```python
from build123d import *

# Parameters (mm, degrees)
SKETCH1_R           = 8.75
SKETCH1_R_2         = 6.75
BOSS_EXTRUDE1_DEPTH = 5.25
SKETCH2_R           = 10.25
SKETCH2_R_2         = 6.75
BOSS_EXTRUDE2_DEPTH = 1
CHAMFER1_SIZE       = 1.050311307
CHAMFER1_SIZE_2     = 1.5
CHAMFER2_SIZE       = 1
CHAMFER3_SIZE       = 0.5


with BuildPart() as part:
    # Sketch1 → Boss-Extrude1 (new, symmetric)
    with BuildSketch(Plane.XY):
        with Locations(Location((0, 0, 0), (0, 0, 180))):
            Circle(SKETCH1_R)
        with Locations(Location((0, 0, 0), (0, 0, 180))):
            Circle(SKETCH1_R_2, mode=Mode.SUBTRACT)
    extrude(amount=BOSS_EXTRUDE1_DEPTH, both=True)

    # Sketch2 → Boss-Extrude2 (add)
    with BuildSketch(Plane.XY.offset(5.25)):
        Circle(SKETCH2_R)
        with Locations(Location((0, 0, 0), (0, 0, 180))):
            Circle(SKETCH2_R_2, mode=Mode.SUBTRACT)
    boss_extrude2 = extrude(amount=BOSS_EXTRUDE2_DEPTH)

    # Mirror1: Boss-Extrude2 across plane
    add(boss_extrude2.mirror(Plane.XY))

    # Chamfer1
    # the kernel refuses this chamfer: 1.5, 1.050311307 mm, written as the material it adds along each edge
    with BuildSketch(Plane(origin=(0, 0, -5.25), x_dir=(-1, 0, 0), z_dir=(0, 1, 0))) as chamfer1_piece_1_section:
        Polygon((8.75, CHAMFER1_SIZE), (8.75 + CHAMFER1_SIZE_2, 0), (8.75, 0), align=None)
    chamfer1_piece_1 = revolve(axis=Axis((0, 0, -5.25), (0, 0, 1)), mode=Mode.PRIVATE)
    chamfer1_piece_1 = chamfer1_piece_1 & Plane(origin=(0, 0, -4.738052243), x_dir=(1, 0, 0), z_dir=(0, 0, 1)) * Cylinder(10.25, 42, mode=Mode.PRIVATE)
    add(chamfer1_piece_1)
    with BuildSketch(Plane(origin=(0, 0, 5.25), x_dir=(-1, 0, 0), z_dir=(0, 1, 0))) as chamfer1_piece_2_section:
        Polygon((8.75, -CHAMFER1_SIZE), (8.75 + CHAMFER1_SIZE_2, 0), (8.75, 0), align=None)
    chamfer1_piece_2 = revolve(axis=Axis((0, 0, 5.25), (0, 0, 1)), mode=Mode.PRIVATE)
    chamfer1_piece_2 = chamfer1_piece_2 & Plane(origin=(0, 0, 4.738052243), x_dir=(1, 0, 0), z_dir=(0, 0, -1)) * Cylinder(10.25, 42, mode=Mode.PRIVATE)
    add(chamfer1_piece_2)

    # Chamfer2
    chamfer2_edges = [part.edges().sort_by_distance(p)[0] for p in [
        (6.75, 0, 6.25),
        (6.75, 0, -6.25),
    ]]
    chamfer(chamfer2_edges, length=CHAMFER2_SIZE)

    # Chamfer3
    chamfer3_edges = [part.edges().sort_by_distance(p)[0] for p in [
        (-10.25, 0, 6.25),
        (-10.25, 0, -6.25),
    ]]
    chamfer(chamfer3_edges, length=CHAMFER3_SIZE)


solid = part.part
```
Design review of the part built by this model. Coordinates are the model's own, in mm. A direction names the side the tool comes from. Round coordinates to 2 decimals unless told otherwise and drop trailing zeros. Order: outer loops, then holes, each group sorted by start corner. A loop starts at its lowest first (then second) coordinate and runs counter-clockwise, first axis right, second up. Notation, with made-up numbers: M 78.5,40 L 111.5,40 A13 ccw 111.5,60 Z; hole C 70.5,53 d4. An arc over 180 degrees is marked long. Put each result on its own line as item: value.
Q1. Draft analysis for pull direction X (two halves, no side actions). For faces 1 (the face through (-7, -4, 6.25)), 2 (the face through (1.46, 6.59, 0.07)), 3 (the face through (-2.222, -10.006, -5.496)), state which applies: released by +X, released by -X, zero draft, split by the parting line, or undercut.
Reported:
face 1: zero draft
face 2: undercut
face 3: split by the parting line
Q2. Machinability: for faces 4 (the face through (-2.222, -10.006, 5.496)), 5 (the face through (1.9, 8.54, 0.06)), which of the approach directions +Z, -Z, +X, -X, +Y, -Y give a long, thin tool a straight path to every point of the face, cutting with its end or side? Answer none if there is none.
Reported:
face 4: +Z, -Z
face 5: none
Q3. To check wall thickness, follow line 1 (Y direction, x = 0, z = -0.75); line 2 (X direction, y = 1.75, z = -2.25); line 3 (Y direction, x = 7, z = 2). State the ranges of each line that lie inside material, in increasing order.
Reported:
line 1: -8.75 to -6.75, 6.75 to 8.75
line 2: -8.57 to -6.52, 6.52 to 8.57
line 3: -5.25 to 5.25
Q4. Consider section A-A (y = 0). State the section outline as (x, z) points, and give its area (3 significant figures).
Reported:
outline: M -10.25,-5.75 L -9.75,-6.25 L -7.75,-6.25 L -6.75,-5.25 L -6.75,5.25 L -7.75,6.25 L -9.75,6.25 L -10.25,5.75 L -10.25,5.25 L -8.75,4.2 L -8.75,-4.2 L -10.25,-5.25 Z; M 6.75,-5.25 L 7.75,-6.25 L 9.75,-6.25 L 10.25,-5.75 L 10.25,-5.25 L 8.75,-4.2 L 8.75,4.2 L 10.25,5.25 L 10.25,5.75 L 9.75,6.25 L 7.75,6.25 L 6.75,5.25 Z
area: 56.7 mm²
Q5. Insertion check: pin 1 Ø6 at (x, y) = (7.5, 7.5) entering from -Z; pin 2 Ø6 at (x, z) = (3.5, 4.5) entering from -Y; pin 3 Ø3 at (y, z) = (6.5, -1.5) entering from +X; pin 4 Ø1 at (x, z) = (0, 2.5) entering from -Y. Each pin has a flat end and moves straight along its axis. Give the tip position at first contact, or say it passes through.
Reported:
pin 1: z = -6.25
pin 2: y = -10.23
pin 3: x = 7.18
pin 4: y = -8.75
Q6. Consider section C-C (z = 3.25). State the section outline as (x, y) points, and give its area (3 significant figures).
Reported:
outline: C 0,0 d17.5; hole C 0,0 d13.5
area: 97.4 mm²
